Geometry check sheet. Reference: the model listing, model coordinates, mm. Coordinates: 2 decimals unless noted, no trailing zeros. Write each loop counter-clockwise with the first axis right and the second up, starting at its lowest first coordinate (ties: lowest second). Pieces come first, ordered by that corner, then holes. Notation, with made-up numbers: (48, 36) -> (62, 36) arc R19 cw to (62, 42) -> close; hole circle Ø11 at (29.25, -1). An arc over 180 degrees is marked (long way). Answer in a Markdown table with one row per item. Add a question column.
Q1. Section check B-B, the plane y = -132. Record the boundary of the cut face in (x, z), and give its area (3 significant figures).
Q2. Section check A-A, the plane z = -780.5. Record the boundary of the cut face in (x, y).
Q3. Section check C-C, the plane x = 725.5. Record the boundary of the cut face in (y, z), and give its area (3 significant figures).
Q4. Gauge pin test, flat ends, axial feed: P1, Ø2, axis at x = 270, y = -164.5, coming from the -Z side; P2, Ø11.5, axis at x = -7.5, z = -472.5, coming from the -Y side. Record the tip position at first contact, or that the pin passes through.
Q5. Thickness scan on line 1 (X direction, y = -321, z = -95); line 2 (Z direction, x = -392, y = 68). Record the ranges inside material, lowest first.
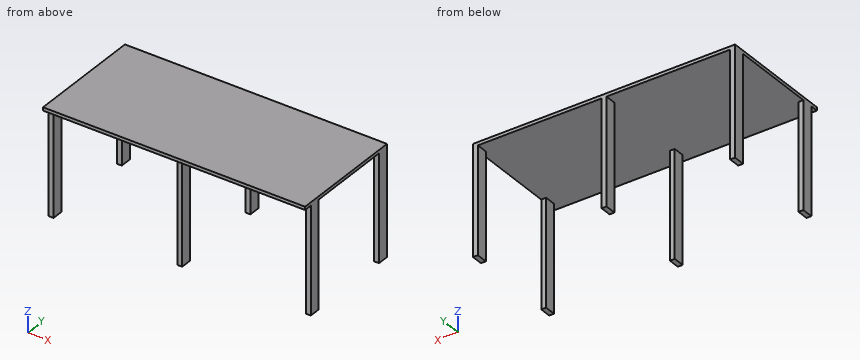
```python
from build123d import *

# Parameters (mm, degrees)
F0_W     = 2057.4
F0_H     = 914.4
F1_DEPTH = 863.6
F2_W     = 63.5
F2_H     = 838.2
F2_W_2   = 673.1
F3_DEPTH = 2057.401
F4_W     = 971.55
F4_H     = 838.2
F5_DEPTH = 850.901


with BuildPart() as f1:
    # F0 (on Top) → F1 (new body)
    with BuildSketch(Plane.XY):
        Rectangle(F0_W, F0_H)
    extrude(amount=-F1_DEPTH)

    # F2 (on face) → F3 (cut, through all)
    with BuildSketch(Plane.YZ.offset(1028.7)):
        with Locations((-425.45, -444.5)):
            Rectangle(F2_W, F2_H)
        with Locations((31.75, -444.5)):
            Rectangle(F2_W_2, F2_H)
    extrude(amount=-F3_DEPTH, mode=Mode.SUBTRACT)

    # F4 (on face) → F5 (cut, through all)
    with BuildSketch(Plane.XZ.offset(393.7)):
        with Locations((-504.825, -444.5)):
            Rectangle(F4_W, F4_H)
        with Locations((504.825, -444.5)):
            Rectangle(F4_W, F4_H)
    extrude(amount=-F5_DEPTH, mode=Mode.SUBTRACT)


solid = f1.part
```
Calculated:
| question | item | result |
|---|---|---|
| 1 | outline | (-1028.7, -25.4) -> (1028.7, -25.4) -> (1028.7, 0) -> (-1028.7, 0) -> close |
| 1 | area | 52,300 mm² |
| 2 | outline | (-1028.7, -393.7) -> (-990.6, -393.7) -> (-990.6, -304.8) -> (-1028.7, -304.8) -> close; (-1028.7, 368.3) -> (-990.6, 368.3) -> (-990.6, 457.2) -> (-1028.7, 457.2) -> close; (-19.05, -393.7) -> (19.05, -393.7) -> (19.05, -304.8) -> (-19.05, -304.8) -> close; (-19.05, 368.3) -> (19.05, 368.3) -> (19.05, 457.2) -> (-19.05, 457.2) -> close; (990.6, -393.7) -> (1028.7, -393.7) -> (1028.7, -304.8) -> (990.6, -304.8) -> close; (990.6, 368.3) -> (1028.7, 368.3) -> (1028.7, 457.2) -> (990.6, 457.2) -> close |
| 3 | outline | (-457.2, -25.4) -> (457.2, -25.4) -> (457.2, 0) -> (-457.2, 0) -> close |
| 3 | area | 23,200 mm² |
| 4 | P1 | stops at z = -25.4 |
| 4 | P2 | stops at y = -393.7 |
| 5 | line 1 | x = -1028.7 to -990.6, -19.05 to 19.05, 990.6 to 1028.7 |
| 5 | line 2 | z = -25.4 to 0 |
